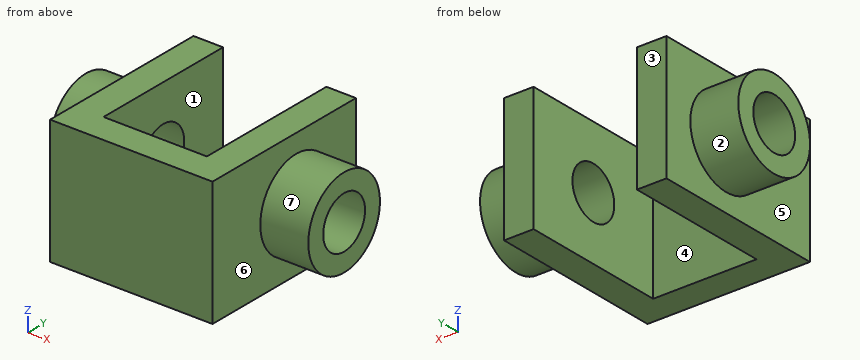
```python
from build123d import *

# Parameters (mm, degrees)
BOSS_EXTRUDE1_DEPTH = 34
SKETCH2_R           = 12
SKETCH2_R_2         = 7
BOSS_EXTRUDE3_DEPTH = 13
BOSS_EXTRUDE5_START = -21
SKETCH4_R           = 12
SKETCH4_R_2         = 7
BOSS_EXTRUDE5_DEPTH = 21
SKETCH9_R           = 7
CUT_EXTRUDE1_DEPTH  = 8
CUT_EXTRUDE2_START  = -8
SKETCH10_R          = 7
CUT_EXTRUDE2_DEPTH  = 8


with BuildPart() as part:
    # Sketch1 → Boss-Extrude1 (new body)
    with BuildSketch(Plane.XY):
        Polygon((0, 0), (44, 0), (44, 48), (36, 48), (36, 8), (8, 8), (8, 48), (0, 48), align=None)
    extrude(amount=-BOSS_EXTRUDE1_DEPTH)

    # Sketch2 → Boss-Extrude3 (add)
    with BuildSketch(Plane.ZY):
        with Locations(Location((-17, 28, 0), (0, 0, 90))):
            Circle(SKETCH2_R)
        with Locations(Location((-17, 28, 0), (0, 0, 90))):
            Circle(SKETCH2_R_2, mode=Mode.SUBTRACT)
    extrude(amount=BOSS_EXTRUDE3_DEPTH)

    # Sketch4 → Boss-Extrude5 (add)
    with BuildSketch(Plane.ZY.offset(-36).offset(BOSS_EXTRUDE5_START)):
        with Locations(Location((-17, 28, 0), (0, 0, 90))):
            Circle(SKETCH4_R)
        with Locations(Location((-17, 28, 0), (0, 0, 90))):
            Circle(SKETCH4_R_2, mode=Mode.SUBTRACT)
    extrude(amount=BOSS_EXTRUDE5_DEPTH)

    # Sketch9 → Cut-Extrude1 (cut)
    with BuildSketch(Plane(origin=(44, 0, 0), x_dir=(0, 0, -1), z_dir=(1, 0, 0))):
        with Locations(Location((17, 28, 0), (0, 0, 90))):
            Circle(SKETCH9_R)
    extrude(amount=-CUT_EXTRUDE1_DEPTH, mode=Mode.SUBTRACT)

    # Sketch10 → Cut-Extrude2 (cut)
    with BuildSketch(Plane.ZY.offset(CUT_EXTRUDE2_START)):
        with Locations(Location((-17, 28, 0), (0, 0, 90))):
            Circle(SKETCH10_R)
    extrude(amount=CUT_EXTRUDE2_DEPTH, mode=Mode.SUBTRACT)


solid = part.part
```
For this review, take the finished solid that the model builds, in its own axes (mm). Face numbers are marked on the shaded views. A direction names the side the tool comes from. Round coordinates to 2 decimals unless told otherwise and drop trailing zeros. Order: outer loops, then holes, each group sorted by start corner. A loop starts at its lowest first (then second) coordinate and runs counter-clockwise, first axis right, second up. Notation, with made-up numbers: (-32, -25) -> (22, -25) arc R31 ccw to (22, 7) -> close; hole circle Ø9 at (-8, 35.25). An arc over 180 degrees is marked (long way). Use a Markdown table: item, result.
Item 1: Take a section at D-D (y = 42). State the section outline as (x, z) points.
Resolved:
| item | result |
|---|---|
| outline | (0, -34) -> (8, -34) -> (8, 0) -> (0, 0) -> close; (36, -34) -> (44, -34) -> (44, 0) -> (36, 0) -> close |
Item 2: Take a section at B-B (z = -17). State the section outline as (x, y) points.
Resolved:
| item | result |
|---|---|
| outline | (-13, 16) -> (0, 16) -> (0, 0) -> (44, 0) -> (44, 16) -> (57, 16) -> (57, 21) -> (36, 21) -> (36, 8) -> (8, 8) -> (8, 21) -> (-13, 21) -> close; (-13, 35) -> (8, 35) -> (8, 48) -> (0, 48) -> (0, 40) -> (-13, 40) -> close; (36, 35) -> (57, 35) -> (57, 40) -> (44, 40) -> (44, 48) -> (36, 48) -> close |
Item 3: Machinability: for the marked faces 1, 2 and 3, which of the approach directions +Z, -Z, +X, -X, +Y, -Y give a long, thin tool a straight path to every point of the face, cutting with its end or side? Answer none if there is none.
Resolved:
| item | result |
|---|---|
| face 1 | +Z, -Z, +Y |
| face 2 | -X |
| face 3 | +Z, -Z, +X, -X, +Y |
Item 4: Take a section at A-A (y = 28). State the section outline as (x, z) points, plus the area to 3 significant figures.
Resolved:
| item | result |
|---|---|
| outline | (-13, -29) -> (0, -29) -> (0, -34) -> (8, -34) -> (8, -24) -> (-13, -24) -> close; (-13, -10) -> (8, -10) -> (8, 0) -> (0, 0) -> (0, -5) -> (-13, -5) -> close; (36, -34) -> (44, -34) -> (44, -29) -> (57, -29) -> (57, -24) -> (36, -24) -> close; (36, -10) -> (57, -10) -> (57, -5) -> (44, -5) -> (44, 0) -> (36, 0) -> close |
| area | 580 mm² |
Item 5: Take a section at C-C (x = 42). State the section outline as (y, z) points, plus the area to 3 significant figures.
Resolved:
| item | result |
|---|---|
| outline | (0, -34) -> (48, -34) -> (48, 0) -> (0, 0) -> close; hole circle Ø14 at (28, -17) |
| area | 1,480 mm² |
Item 6: For line 1 along Z through (x, y) = (41, 28); line 2 along X through (y, z) = (11.5, -10.5); line 3 along Z through (x, y) = (-8, 28), list the stretches that pass through material, from the lowest coordinate up. Write a range as [from, to].
Resolved:
| item | result |
|---|---|
| line 1 | z = [-34, -24], [-10, 0] |
| line 2 | x = [0, 8], [36, 44] |
| line 3 | z = [-29, -24], [-10, -5] |
Item 7: For pin 1 (8 mm diameter, centred on y = 29, z = -5, fed in from -X); pin 2 (5 mm diameter, centred on y = 12, z = -26.5, fed in from -X), all flat-tipped, find the tip position at first contact; note any pin that passes through.
Resolved:
| item | result |
|---|---|
| pin 1 | stops at x = -13 |
| pin 2 | stops at x = 0 |
Item 8: Draft analysis for pull direction X (two halves, no side actions). For the marked faces 4, 5, 6 and 7, state which applies: +X half, -X half, draft (parallel to the pull), parting line (faces both ways), or undercut.
Resolved:
| item | result |
|---|---|
| face 4 | undercut |
| face 5 | -X half |
| face 6 | +X half |
| face 7 | draft |
